```python
from build123d import *

# Parameters (mm, degrees)
EXTRUDE_1_DEPTH = 1.5
SKETCH_1_4_R    = 1.3
EXTRUDE_2_DEPTH = 9


with BuildPart() as part:
    # Sketch 1 → Extrude 1 (new body)
    with BuildSketch(Plane.XY):
        with BuildLine():
            ThreePointArc((3.188454535, 4.481490565), (2.570411742, 5.19430182), (2.347892547, 6.111123497))
            Line((2.347892547, 6.111123497), (2.347892547, 8.652107453))
            ThreePointArc((2.347892547, 8.652107453), (0, 6.304214905), (-2.347892547, 8.652107453))
            Line((-2.347892547, 8.652107453), (-2.347892547, 6.111123497))
            ThreePointArc((-2.347892547, 6.111123497), (-2.570411742, 5.19430182), (-3.188454535, 4.481490565))
            ThreePointArc((-3.188454535, 4.481490565), (-5.5, 0), (-3.188454535, -4.481490565))
            ThreePointArc((-3.188454535, -4.481490565), (-2.570411742, -5.19430182), (-2.347892547, -6.111123497))
            Line((-2.347892547, -6.111123497), (-2.347892547, -8.652107453))
            ThreePointArc((-2.347892547, -8.652107453), (0, -6.304214905), (2.347892547, -8.652107453))
            Line((2.347892547, -8.652107453), (2.347892547, -6.111123497))
            ThreePointArc((2.347892547, -6.111123497), (2.570411742, -5.19430182), (3.188454535, -4.481490565))
            ThreePointArc((3.188454535, -4.481490565), (5.5, 0), (3.188454535, 4.481490565))
        make_face()
        with BuildLine():
            ThreePointArc((1.55, -2.75), (0, -4.3), (-1.55, -2.75))
            Line((-1.55, -2.75), (-1.55, -2.271563338))
            ThreePointArc((-1.55, -2.271563338), (-2.75, 0), (-1.55, 2.271563338))
            Line((-1.55, 2.271563338), (-1.55, 2.75))
            ThreePointArc((-1.55, 2.75), (0, 4.3), (1.55, 2.75))
            Line((1.55, 2.75), (1.55, 2.271563338))
            ThreePointArc((1.55, 2.271563338), (2.75, 0), (1.55, -2.271563338))
            Line((1.55, -2.271563338), (1.55, -2.75))
        make_face(mode=Mode.SUBTRACT)
    extrude(amount=EXTRUDE_1_DEPTH)

    # Sketch 1_4 → Extrude 2 (add)
    with BuildSketch(Plane.XY):
        with BuildLine():
            ThreePointArc((-2.347892547, -8.652107453), (0, -11), (2.347892547, -8.652107453))
            ThreePointArc((2.347892547, -8.652107453), (0, -6.304214905), (-2.347892547, -8.652107453))
        make_face()
        with Locations((0, -8.652107453)):
            Circle(SKETCH_1_4_R, mode=Mode.SUBTRACT)
        with BuildLine():
            ThreePointArc((-2.347892547, 8.652107453), (0, 6.304214905), (2.347892547, 8.652107453))
            ThreePointArc((2.347892547, 8.652107453), (0, 11), (-2.347892547, 8.652107453))
        make_face()
        with Locations((0, 8.652107453)):
            Circle(SKETCH_1_4_R, mode=Mode.SUBTRACT)
    extrude(amount=EXTRUDE_2_DEPTH)


solid = part.part
```
Here's how the part is built. I have some questions about the finished solid (model axes, mm). A direction names the side the tool comes from. Round coordinates to 2 decimals unless told otherwise and drop trailing zeros. Loops run counter-clockwise (first coordinate to the right, second up) from the corner with the lowest first, then second, coordinate; pieces in that order, holes last. Notation, with made-up numbers: (41, 45.5) -> (76, 45.5) arc R19 ccw to (76, 56.5) -> close; hole circle Ø9 at (-4.75, 61.25). An arc over 180 degrees is marked (long way). Answer as CSV lines item,"result".
1. If I drill on L1, parallel to Y at x = 0, z = 3.75; L2, parallel to X at y = 6.75, z = 1; L3, parallel to Y at x = 1, z = 2, over which ranges is the centre line in solid material (lowest first)?
Final values:
L1,"y = -11 to -9.95, -7.35 to -6.3, 6.3 to 7.35, 9.95 to 11"
L2,"x = -2.35 to 2.35"
L3,"y = -10.78 to -9.48, -7.82 to -6.53, 6.53 to 7.82, 9.48 to 10.78"
2. If we section it at C-C on y = -1.5: Please give me the cut outline in (x, z), plus the area to 3 significant figures.
Final values:
outline,"(-5.29, 0) -> (-2.3, 0) -> (-2.3, 1.5) -> (-5.29, 1.5) -> close; (2.3, 0) -> (5.29, 0) -> (5.29, 1.5) -> (2.3, 1.5) -> close"
area,"8.96 mm^2"
3. If we section it at D-D on y = -8: Please give me the cut outline in (x, z), plus the area to 3 significant figures.
Final values:
outline,"(-2.35, 0) -> (-1.12, 0) -> (-1.12, 9) -> (-2.26, 9) -> (-2.26, 1.5) -> (-2.35, 1.5) -> close; (1.12, 0) -> (2.35, 0) -> (2.35, 1.5) -> (2.26, 1.5) -> (2.26, 9) -> (1.12, 9) -> close"
area,"20.6 mm^2"
4. Which directions (+Z, -Z, +X, -X, +Y, -Y) give clear straight access to the entire face, cutting with the end or side of a thin tool? Please do faces 1 (the face through (0, 4.3, 0.7)), 2 (the face through (-2.348, -7, 1)), 3 (the face through (2.348, 7, 1)), 4 (the face through (-2.348, 7, 1)).
Final values:
face 1,"+Z, -Z"
face 2,"+Z, -Z, -X, -Y"
face 3,"+Z, -Z, +X, +Y"
face 4,"+Z, -Z, -X, +Y"
5. If we section it at B-B on x = 0: Please give me the cut outline in (y, z), plus the area to 3 significant figures.
Final values:
outline,"(-11, 0) -> (-9.95, 0) -> (-9.95, 9) -> (-11, 9) -> close; (-7.35, 0) -> (-4.3, 0) -> (-4.3, 1.5) -> (-6.3, 1.5) -> (-6.3, 9) -> (-7.35, 9) -> close; (4.3, 0) -> (7.35, 0) -> (7.35, 9) -> (6.3, 9) -> (6.3, 1.5) -> (4.3, 1.5) -> close; (9.95, 0) -> (11, 0) -> (11, 9) -> (9.95, 9) -> close"
area,"43.7 mm^2"
6. Thinking about a two-plate mould opening in Y: for faces 5 (the face through (2.75, 0.04, 0.74)), 6 (the face through (2.564, -5.206, 0.74)), 7 (the face through (2.348, -7, 1)), which applies, released by +Y, released by -Y, zero draft, split by the parting line, or undercut?
Final values:
face 5,"undercut"
face 6,"released by -Y"
face 7,"zero draft"
7. For pin 1 (3 mm diameter, centred on y = 4.5, z = 3.5, fed in from -X); pin 2 (1.2 mm diameter, centred on y = -7, z = 0.5, fed in from -X); pin 3 (1.2 mm diameter, centred on y = 7.5, z = 1, fed in from +X); pin 4 (0.5 mm diameter, centred on y = 2.5, z = 0.5, fed in from +X), each with a flat end and sliding along its axis, tell me the tip position at first contact or that it passes through.
Final values:
pin 1,"passes through"
pin 2,"stops at x = -2.35"
pin 3,"stops at x = 2.35"
pin 4,"stops at x = 5.02"
8. If we section it at A-A on z = 8.25: Please give me the cut outline in (x, y), plus the area to 3 significant figures.
Final values:
outline,"circle Ø4.7 at (0, -8.65); circle Ø4.7 at (0, 8.65); hole circle Ø2.6 at (0, -8.65); hole circle Ø2.6 at (0, 8.65)"
area,"24.0 mm^2"
